Geometry check sheet. Reference: drawing and pictorial views, mm from the part's lowest x, y, z. A direction names the side the tool comes from. Coordinates: 2 decimals unless noted, no trailing zeros. Loops run counter-clockwise (first coordinate to the right, second up) from the corner with the lowest first, then second, coordinate; pieces in that order, holes last. Notation, with made-up numbers: (-14.5, 41) - (24.5, 41) arc R21 ccw to (24.5, 75) - close; hole circle Ø11 at (37.25, -19.5). An arc over 180 degrees is marked (long way). One line per item, written item: value.
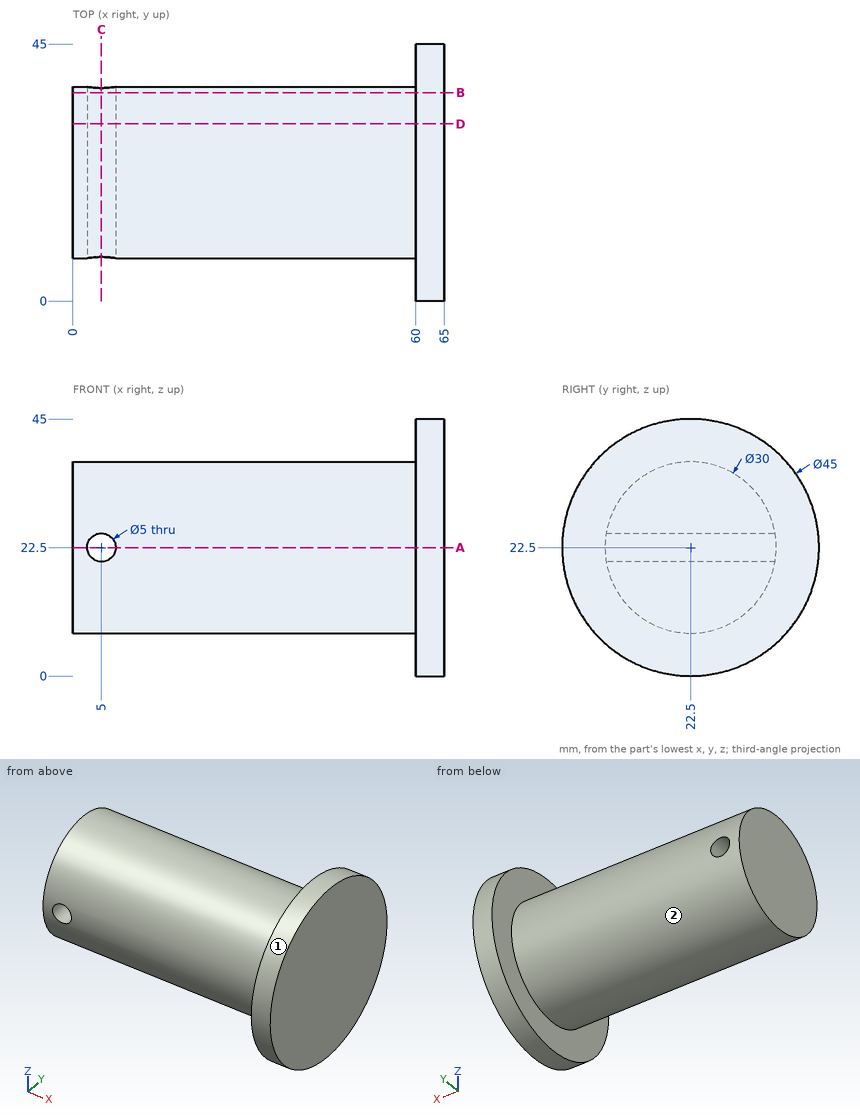
(1) Cross-section at C-C on x = 5. Record the cut outline in (y, z), and give its area (3 significant figures).
Reply:
outline: (7.71, 20) arc R15 ccw to (37.29, 20) - close; (7.71, 25) - (37.29, 25) arc R15 ccw to start
area: 558 mm2
(2) Access from +Z, -Z, +X, -X, +Y, -Y to the whole of each face (thin tool, end or side, straight path). Record for the marked faces 1 and 2.
Reply:
face 1: +X, -X
face 2: -X
(3) Cross-section at D-D on y = 31. Record the cut outline in (x, z), and give its area (3 significant figures).
Reply:
outline: (0, 10.14) - (60, 10.14) - (60, 1.67) - (65, 1.67) - (65, 43.33) - (60, 43.33) - (60, 34.86) - (0, 34.86) - close; hole circle Ø5 at (5, 22.5)
area: 1,670 mm2
(4) Material ranges on probe 1 along X at (y, z) = (15, 22.5); probe 2 along X at (y, z) = (31.5, 37); probe 3 along Z at (x, y) = (25, 9), recorded low to high. Write a range as from..to.
Reply:
probe 1: 0..2.5, 7.5..65
probe 2: 60..65
probe 3: 15.96..29.04
(5) Cross-section at A-A on z = 22.5. Record the cut outline in (x, y), and give its area (4 significant figures).
Reply:
outline: (0, 7.5) - (2.5, 7.5) - (2.5, 37.5) - (0, 37.5) - close; (7.5, 7.5) - (60, 7.5) - (60, 0) - (65, 0) - (65, 45) - (60, 45) - (60, 37.5) - (7.5, 37.5) - close
area: 1,875 mm2
(6) Go/stop test with flat-tipped pins: pin 1 Ø3 at (x, z) = (17, 35.5) entering from +Y; pin 2 Ø2 at (x, z) = (32, 25.5) entering from -Y; pin 3 Ø10 at (x, z) = (42, 39) entering from -Y; pin 4 Ø4 at (x, z) = (5, 22.5) entering from +Y. Record where each tip stops, or that it passes through.
Reply:
pin 1: y = 32.13
pin 2: y = 7.63
pin 3: y = 12.87
pin 4: through
(7) Cross-section at B-B on y = 36.5. Record the cut outline in (x, z), and give its area (3 significant figures).
Reply:
outline: (0, 17.11) - (60, 17.11) - (60, 4.89) - (65, 4.89) - (65, 40.11) - (60, 40.11) - (60, 27.89) - (0, 27.89) - close; hole circle Ø5 at (5, 22.5)
area: 803 mm2
